```python
from build123d import *

# Parameters (mm, degrees)
SKETCH1_R           = 34.9
SKETCH1_R_2         = 29.9
EXTRUDE_THIN1_DEPTH = 10
SKETCH1_3_W         = 5
SKETCH1_3_H         = 69.8
SKETCH1_3_W_2       = 69.8
SKETCH1_3_H_2       = 5
EXTRUDE_THIN2_DEPTH = 10
SKETCH2_W           = 53.342781532
SKETCH2_H           = 5
BOSS_EXTRUDE1_DEPTH = 80
SKETCH3_R           = 1.5621
BOSS_EXTRUDE2_DEPTH = 5
BOSS_EXTRUDE4_DEPTH = 20
EXTRUDE_THIN4_DEPTH = 20


# Read off the part's stored shape, not the designer's step: Extrude-Thin4
with BuildPart() as part:
    # Sketch1 → Extrude-Thin1 (new body)
    with BuildSketch(Plane(origin=(0, 0, 0), x_dir=(1, 0, 0), z_dir=(0, 1, 0))):
        Circle(SKETCH1_R)
        Circle(SKETCH1_R_2, mode=Mode.SUBTRACT)
    extrude(amount=EXTRUDE_THIN1_DEPTH)

    # Sketch1_3 → Extrude-Thin2 (add)
    with BuildSketch(Plane(origin=(0, 0, 0), x_dir=(1, 0, 0), z_dir=(0, 1, 0))):
        Rectangle(SKETCH1_3_W, SKETCH1_3_H)
        Rectangle(SKETCH1_3_W_2, SKETCH1_3_H_2)
    extrude(amount=EXTRUDE_THIN2_DEPTH)

    # Sketch2 → Boss-Extrude1 (add)
    with BuildSketch(Plane(origin=(0, 10, 0), x_dir=(1, 0, 0), z_dir=(0, 1, 0))):
        Rectangle(SKETCH2_W, SKETCH2_H)
    extrude(amount=BOSS_EXTRUDE1_DEPTH)

    # Sketch3 → Boss-Extrude2 (add)
    with BuildSketch(Plane.XY.offset(2.5)):
        with Locations(Location((-9.525, 77.1246, 0), (0, 0, 180))):
            Circle(SKETCH3_R)
        with Locations(Location((-9.525, 20, 0), (0, 0, 180))):
            Circle(SKETCH3_R)
        with Locations(Location((9.525, 20, 0), (0, 0, 180))):
            Circle(SKETCH3_R)
        with Locations(Location((9.525, 77.1246, 0), (0, 0, 180))):
            Circle(SKETCH3_R)
    extrude(amount=BOSS_EXTRUDE2_DEPTH)



with BuildPart() as body_2:
    # Sketch6 → Boss-Extrude4 (new body)
    with BuildSketch(Plane(origin=(0, 90, 0), x_dir=(1, 0, 0), z_dir=(0, 1, 0))):
        with BuildLine():
            Line((0, 30), (0, 34.9))
            ThreePointArc((0, 34.9), (-24.678026663, 24.678026663), (-34.9, 0))
            Line((-34.9, 0), (-30, 0))
            ThreePointArc((-30, 0), (-21.213203436, 21.213203436), (0, 30))
        make_face()
        with BuildLine():
            Line((-30, 0), (-34.9, 0))
            ThreePointArc((-34.9, 0), (-24.678026663, -24.678026663), (0, -34.9))
            Line((0, -34.9), (0, -30))
            ThreePointArc((0, -30), (-21.213203436, -21.213203436), (-30, 0))
        make_face()
        with BuildLine():
            ThreePointArc((0, -34.9), (24.678026663, -24.678026663), (34.9, 0))
            Line((34.9, 0), (30, 0))
            ThreePointArc((30, 0), (21.213203436, -21.213203436), (0, -30))
            Line((0, -30), (0, -34.9))
        make_face()
    extrude(amount=BOSS_EXTRUDE4_DEPTH)


with BuildPart() as part_1:
    add(part.part)

    add(body_2.part)  # Extrude-Thin4 merges body 2
    # Extrude-Thin4 outline → Extrude-Thin4 (add)
    with BuildSketch(Plane(origin=(0, 90, 0), x_dir=(1, 0, 0), z_dir=(0, 1, 0))):
        with BuildLine():
            ThreePointArc((-34.9, -1.61e-07), (-34.877578623, 1.250803494), (-34.81034329, 2.5))
            Line((-34.81034329, 2.5), (-34.9, 2.5))
            Line((-34.9, 2.5), (-34.9, -1.61e-07))
        make_face()
        with BuildLine():
            Line((-2.5, 34.9), (-2.5, 34.81034329))
            ThreePointArc((-2.5, 34.81034329), (-1.250803574, 34.87757862), (0, 34.9))
            Line((0, 34.9), (-2.5, 34.9))
        make_face()
        with BuildLine():
            ThreePointArc((-34.81034329, -2.5), (-34.877578617, -1.250803655), (-34.9, -1.61e-07))
            Line((-34.9, -1.61e-07), (-34.9, -2.5))
            Line((-34.9, -2.5), (-34.81034329, -2.5))
        make_face()
        with BuildLine():
            Line((2.5, 34.9), (0, 34.9))
            Line((0, 34.9), (0, 30))
            ThreePointArc((0, 30), (-1.25108838, 29.973901612), (-2.5, 29.895651858))
            Line((-2.5, 29.895651858), (-2.5, 2.5))
            Line((-2.5, 2.5), (-29.895651858, 2.5))
            ThreePointArc((-29.895651858, 2.5), (-30, 0), (-29.895651858, -2.5))
            Line((-29.895651858, -2.5), (-2.5, -2.5))
            Line((-2.5, -2.5), (-2.5, -29.895651858))
            ThreePointArc((-2.5, -29.895651858), (0, -30), (2.5, -29.895651858))
            Line((2.5, -29.895651858), (2.5, -2.5))
            Line((2.5, -2.5), (29.895651858, -2.5))
            ThreePointArc((29.895651858, -2.5), (29.973901612, -1.25108838), (30, 0))
            Line((30, 0), (34.9, 0))
            Line((34.9, 0), (34.9, 2.5))
            Line((34.9, 2.5), (2.5, 2.5))
            Line((2.5, 2.5), (2.5, 34.9))
        make_face()
        with BuildLine():
            ThreePointArc((0, -34.9), (-1.250803574, -34.87757862), (-2.5, -34.81034329))
            Line((-2.5, -34.81034329), (-2.5, -34.9))
            Line((-2.5, -34.9), (0, -34.9))
        make_face()
        with BuildLine():
            ThreePointArc((2.5, -34.81034329), (1.250803574, -34.87757862), (0, -34.9))
            Line((0, -34.9), (2.5, -34.9))
            Line((2.5, -34.9), (2.5, -34.81034329))
        make_face()
        with BuildLine():
            ThreePointArc((34.9, 0), (34.87757862, -1.250803574), (34.81034329, -2.5))
            Line((34.81034329, -2.5), (34.9, -2.5))
            Line((34.9, -2.5), (34.9, 0))
        make_face()
    extrude(amount=EXTRUDE_THIN4_DEPTH)


solid = part_1.part
```
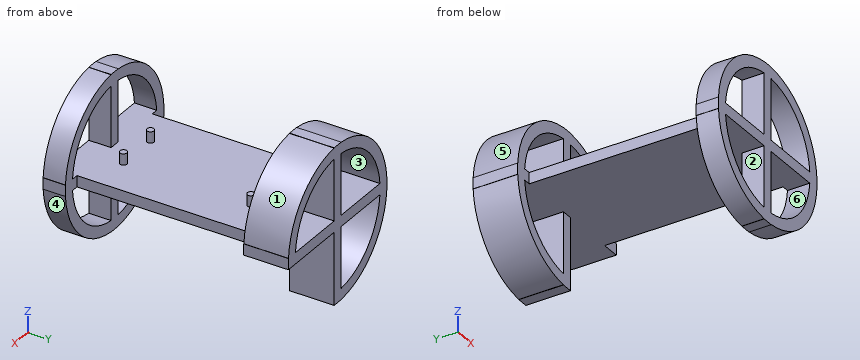
Geometry check sheet. Reference: the model listing, model coordinates, mm. Face numbers are marked on the shaded views. A direction names the side the tool comes from. Round coordinates to 2 decimals unless told otherwise and drop trailing zeros. Loops run counter-clockwise (first coordinate to the right, second up) from the corner with the lowest first, then second, coordinate; pieces in that order, holes last. Notation, with made-up numbers: M -12,53 L 17,53 A20 cw 17,77 Z; hole C -32,30.25 d3. An arc over 180 degrees is marked long. Return JSON: item names as keys, results as strings. Group by question number.
(1) Scan lines: line 1 along Y through (x, z) = (0, 13); line 2 along Z through (x, y) = (-20, 88); line 3 along Y through (x, z) = (11.5, -30). Record each from-to range of solid material in increasing order. Write a range as [from, to].
(2) Set-up check for the marked faces 1, 2 and 3: record each of +Z, -Z, +X, -X, +Y, -Y from which the full face is reachable in a straight line by a thin tool's end or side.
(3) Go/stop test with flat-tipped pins: pin 1 (8 mm diameter, centred on y = 4, z = -13, fed in from -X); pin 2 (8 mm diameter, centred on y = 7, z = 17, fed in from +X); pin 3 (5.5 mm diameter, centred on y = 69, z = -1, fed in from +X). Record where each tip stops, or that it passes through.
(4) Mould release check, pull along X, two halves, no side actions. Record for the marked faces 4, 5 and 6: pulls with the +X half, pulls with the -X half, needs draft (parallel to the pull), parting line crosses it, or undercut.
(5) Section check C-C, the plane x = 0.5. Enter the section's corners in (y, z).
(6) Section check B-B, the plane z = -26. Enter the section's corners in (x, y), and give its area (3 significant figures).
(7) Section check A-A, the plane y = 103.5. Enter the section's corners in (x, z).
(8) Section check D-D, the plane x = -16.5. Enter the section's corners in (y, z), and give its area (3 significant figures).
Data:
{
 "1": {"line 1": "[0, 10], [90, 110]", "line 2": "[-2.5, 2.5]", "line 3": "[0, 10]"},
 "2": {"face 1": "+Z, +X, +Y, -Y", "face 2": "+Y, -Y", "face 3": "+Y"},
 "3": {"pin 1": "x = -33.72", "pin 2": "x = 32.39", "pin 3": "x = 26.67"},
 "4": {"face 4": "pulls with the +X half", "face 5": "pulls with the -X half", "face 6": "undercut"},
 "5": {"outline": "M 0,-34.9 L 10,-34.9 L 10,-2.5 L 90,-2.5 L 90,-34.9 L 110,-34.9 L 110,34.9 L 90,34.9 L 90,2.5 L 10,2.5 L 10,34.9 L 0,34.9 Z"},
 "6": {"outline": "M -23.28,0 L -14.77,0 L -14.77,10 L -23.28,10 Z; M -23.28,90 L -14.97,90 L -14.97,110 L -23.28,110 Z; M -2.5,0 L 2.5,0 L 2.5,10 L -2.5,10 Z; M -2.5,90 L 2.5,90 L 2.5,110 L -2.5,110 Z; M 14.77,0 L 23.28,0 L 23.28,10 L 14.77,10 Z", "area": "487 mm²"},
 "7": {"outline": "M -34.9,-2.5 L -34.81,-2.5 A34.9 ccw -2.5,-34.81 L -2.5,-34.9 L 2.5,-34.9 L 2.5,-2.5 L 34.9,-2.5 L 34.9,2.5 L 34.81,2.5 A34.9 ccw 2.5,34.81 L 2.5,34.9 L -2.5,34.9 L -2.5,34.81 A34.9 ccw -34.81,2.5 L -34.9,2.5 Z; hole M -29.9,-2.5 A30 ccw -2.5,-29.9 L -2.5,-2.5 Z; hole M -29.9,2.5 L -2.5,2.5 L -2.5,29.9 A30 ccw Z; hole M 2.5,2.5 L 29.9,2.5 A30 ccw 2.5,29.9 Z"},
 "8": {"outline": "M 0,-30.75 L 10,-30.75 L 10,-24.94 L 0,-24.94 Z; M 0,-2.5 L 110,-2.5 L 110,2.5 L 0,2.5 Z; M 0,24.94 L 10,24.94 L 10,30.75 L 0,30.75 Z; M 90,-30.75 L 110,-30.75 L 110,-25.05 L 90,-25.05 Z; M 90,25.05 L 110,25.05 L 110,30.75 L 90,30.75 Z", "area": "894 mm²"}
}
